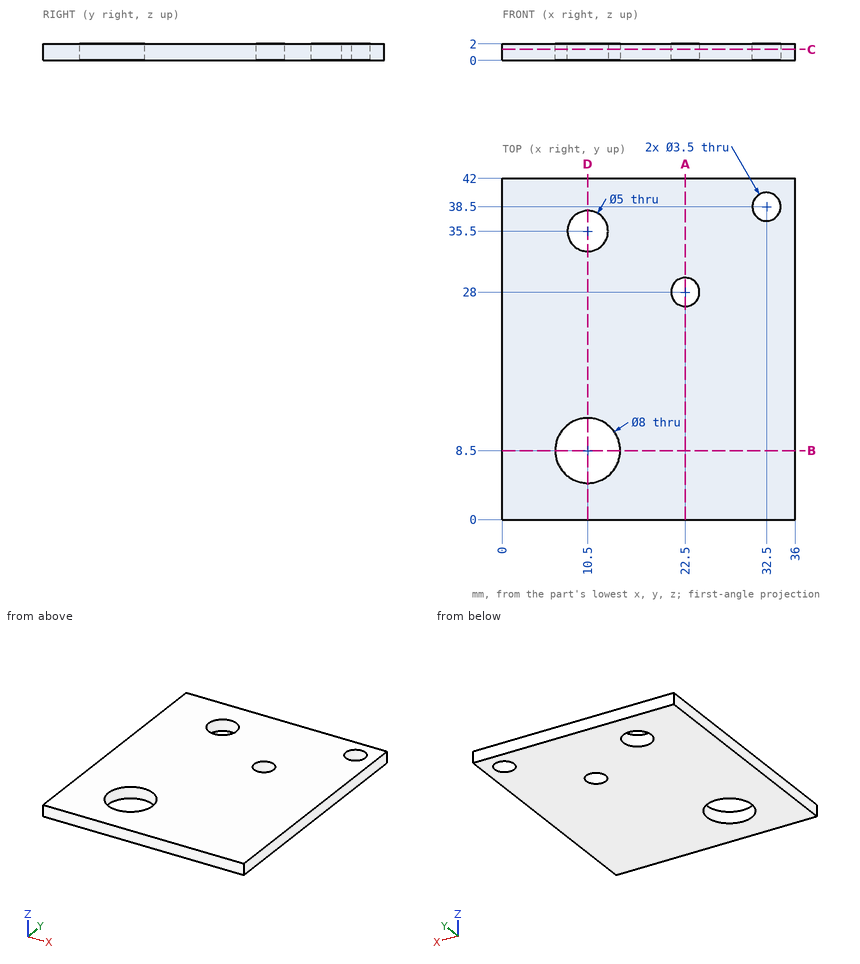
Design review of the part shown in the three views and the two pictorial views. Dimensions are in mm from the part's minimum x, y and z. Round coordinates to 2 decimals unless told otherwise and drop trailing zeros. Write each loop counter-clockwise with the first axis right and the second up, starting at its lowest first coordinate (ties: lowest second). Pieces come first, ordered by that corner, then holes. Notation, with made-up numbers: (23, 58) -> (60, 58) arc R13 cw to (60, 83) -> close; hole circle Ø3 at (66, 47). An arc over 180 degrees is marked (long way). Answer as a JSON object with one key per item and string values.
1. We need section B-B on y = 8.5. State the section outline as (x, z) points.
Results found:
{"outline": "(0, 0) -> (6.5, 0) -> (6.5, 2) -> (0, 2) -> close; (14.5, 0) -> (36, 0) -> (36, 2) -> (14.5, 2) -> close"}
2. To check wall thickness, follow line 1 along X through (y, z) = (37, 1.65); line 2 along Y through (x, z) = (10.5, 0.85); line 3 along Y through (x, z) = (11.5, 1.95). State the ranges of each line that lie inside material, in increasing order.
Results found:
{"line 1": "x = 0 to 8.5, 12.5 to 31.6, 33.4 to 36", "line 2": "y = 0 to 4.5, 12.5 to 33, 38 to 42", "line 3": "y = 0 to 4.63, 12.37 to 33.21, 37.79 to 42"}
3. We need section A-A on x = 22.5. State the section outline as (y, z) points, and give its area (3 significant figures).
Results found:
{"outline": "(0, 0) -> (26.25, 0) -> (26.25, 2) -> (0, 2) -> close; (29.75, 0) -> (42, 0) -> (42, 2) -> (29.75, 2) -> close", "area": "77.0 mm^2"}
4. Clearance check with flat-ended pins moving along their axes: pin 1 (7 mm diameter, centred on x = 10.5, y = 8.5, fed in from -Z); pin 2 (1.5 mm diameter, centred on x = 21, y = 14, fed in from -Z). State where each tip first meets the part, or that it passes through.
Results found:
{"pin 1": "passes through", "pin 2": "stops at z = 0"}
5. We need section D-D on x = 10.5. State the section outline as (y, z) points.
Results found:
{"outline": "(0, 0) -> (4.5, 0) -> (4.5, 2) -> (0, 2) -> close; (12.5, 0) -> (33, 0) -> (33, 2) -> (12.5, 2) -> close; (38, 0) -> (42, 0) -> (42, 2) -> (38, 2) -> close"}
6. We need section C-C on z = 1.35. State the section outline as (x, y) points.
Results found:
{"outline": "(0, 0) -> (36, 0) -> (36, 42) -> (0, 42) -> close; hole circle Ø8 at (10.5, 8.5); hole circle Ø5 at (10.5, 35.5); hole circle Ø3.5 at (22.5, 28); hole circle Ø3.5 at (32.5, 38.5)"}
